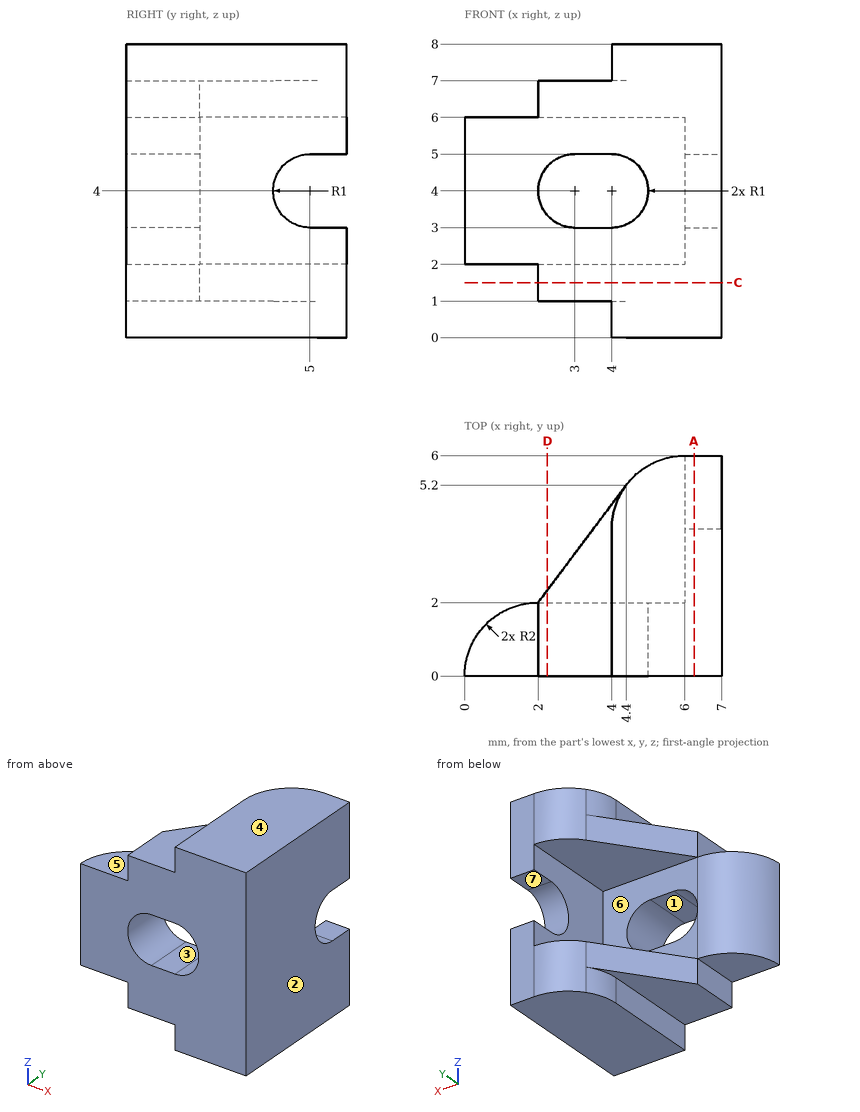
Geometry check sheet. Reference: drawing and pictorial views, mm from the part's lowest x, y, z. A direction names the side the tool comes from. Round coordinates to 2 decimals unless told otherwise and drop trailing zeros. Order: outer loops, then holes, each group sorted by start corner. A loop starts at its lowest first (then second) coordinate and runs counter-clockwise, first axis right, second up. Notation, with made-up numbers: (-18, 26) - (40, 26) arc R26 ccw to (40, 60) - close; hole circle Ø1 at (65.25, 71.25). An arc over 180 degrees is marked (long way). One line per question, with ' | ' between items. Start each with the question number.
(1) Sectioned sample at C-C on z = 1.5. Record the cut outline in (x, y).
(2) Depth check by flat-ended pin: pin 1 Ø1.2 at (y, z) = (3.5, 5) entering from -X; pin 2 Ø2 at (x, y) = (2.5, 1) entering from -Z; pin 3 Ø1.6 at (x, y) = (1, 1) entering from -Z. Enter the tip coordinate at first touch or a pass-through.
(3) Access from +Z, -Z, +X, -X, +Y, -Y to the whole of each face (thin tool, end or side, straight path). Record for the marked faces 5, 6 and 7.
(4) Thickness scan on L1, parallel to Z at x = 6.25, y = 5.8; L2, parallel to Z at x = 4.5, y = 3.05; L3, parallel to Z at x = 1.75, y = 1.45. Record the ranges inside material, lowest first. Write a range as [from, to].
(5) Sectioned sample at D-D on x = 2.25. Record the cut outline in (y, z), and give its area (3 significant figures).
(6) Release check for a two-part mould opening along X. For the marked faces 1, 2, 3 and 4 record: released by +X, released by -X, zero draft, split by the parting line, or undercut.
(7) Sectioned sample at A-A on x = 6.25. Record the cut outline in (y, z), and give its area (3 significant figures).
Conclusion:
1) outline: (2, 0) - (7, 0) - (7, 6) - (6, 6) arc R2 ccw to (4.4, 5.2) - (2, 2) - close
2) pin 1: stops at x = 6 | pin 2: stops at z = 1 | pin 3: stops at z = 2
3) face 5: +Z, -X, +Y, -Y | face 6: -X, +Y | face 7: +X, -X, +Y
4) L1: z = [0, 3], [5, 8] | L2: z = [0, 2], [6, 8] | L3: z = [2, 6]
5) outline: (0, 1) - (2.33, 1) - (2.33, 2) - (2, 2) - (2, 3.34) - (0, 3.34) - close; (0, 4.66) - (2, 4.66) - (2, 6) - (2.33, 6) - (2.33, 7) - (0, 7) - close | area: 10.0 mm2
6) face 1: undercut | face 2: released by +X | face 3: undercut | face 4: zero draft
7) outline: (0, 0) - (6, 0) - (6, 3) - (5, 3) arc R1 cw to (5, 5) - (6, 5) - (6, 8) - (0, 8) - close | area: 44.4 mm2
